Input: dimensioned drawing with shaded views. Units: mm. Origin: part minimum x, y, z. A direction names the side the tool comes from. Round coordinates to 2 decimals unless told otherwise and drop trailing zeros. Order: outer loops, then holes, each group sorted by start corner. A loop starts at its lowest first (then second) coordinate and runs counter-clockwise, first axis right, second up. Notation, with made-up numbers: M 34.5,-36.75 L 46.5,-36.75 A23 cw 46.5,-15.75 Z; hole C 37,-22.75 d6. An arc over 180 degrees is marked long. Use CSV: the item, a comma, the result in double quotes. Start each with the question number.
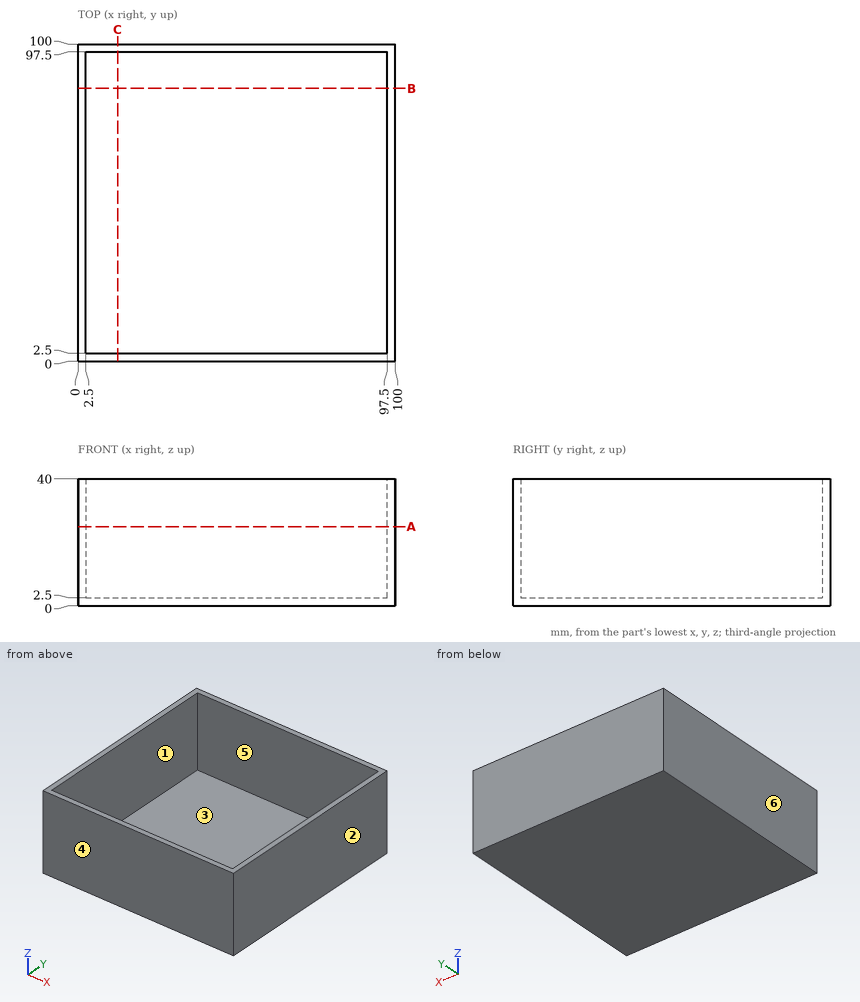
(1) Section B-B on y = 86. Return loops of the section in (x, z).
(2) Line query: line 1 along X through (y, z) = (56, 9.5); line 2 along Z through (x, y) = (46.5, 80.5). Output: solid intervals per line, ascending.
(3) Draft query along Y for the marked faces 1, 2, 3 and 4. Return one class per face: pulls with the +Y half, pulls with the -Y half, needs draft (parallel to the pull), parting line crosses it, or undercut.
(4) Reachability of the marked faces 5 and 6 from +Z, -Z, +X, -X, +Y, -Y: full face, straight path, thin tool, end or side. Return the list, or none.
(5) Section A-A on z = 25. Return loops of the section in (x, y).
(6) Contact query for a flat-ended pin moving along its axis: P1, Ø6, axis at x = 36.5, y = 39, coming from the +Z side. Output: stop coordinate, or through.
Results below:
1,outline,"M 0,0 L 100,0 L 100,40 L 97.5,40 L 97.5,2.5 L 2.5,2.5 L 2.5,40 L 0,40 Z"
2,line 1,"x = 0 to 2.5, 97.5 to 100"
2,line 2,"z = 0 to 2.5"
3,face 1,"undercut"
3,face 2,"needs draft"
3,face 3,"undercut"
3,face 4,"pulls with the -Y half"
4,face 5,"+Z"
4,face 6,"+Z, -Z, -X, +Y, -Y"
5,outline,"M 0,0 L 100,0 L 100,100 L 0,100 Z; hole M 2.5,2.5 L 97.5,2.5 L 97.5,97.5 L 2.5,97.5 Z"
6,P1,"stops at z = 2.5"
